from build123d import *

# Parameters (mm, degrees)
SKICA1_W                 = 150
SKICA1_H                 = 35
P_IDAT_VYSUNUT_M2_DEPTH  = 3
SKICA2_W                 = 6.5
SKICA2_H                 = 11.5
SKICA2_W_2               = 5
SKICA2_H_2               = 10
P_IDAT_VYSUNUT_M3_DEPTH  = 2
SKICA4_W                 = 20
SKICA4_H                 = 5
ODEBRAT_VYSUNUT_M1_DEPTH = 2
SKICA5_W                 = 150
SKICA5_H                 = 5.2
ODEBRAT_VYSUNUT_M3_DEPTH = 1
SKICA7_R                 = 2
ODEBRAT_VYSUNUT_M4_DEPTH = 5
SKICA8_W                 = 8
SKICA8_H                 = 6
P_IDAT_VYSUNUT_M4_DEPTH  = 30
ZAOBLIT1_R               = 1
SKICA9_W                 = 134
SKICA9_H                 = 1
P_IDAT_VYSUNUT_M5_DEPTH  = 4
ZAOBLIT2_R               = 1


with BuildPart() as part:
    # Skica1 → Přidat vysunutím2 (new body)
    with BuildSketch(Plane.XY):
        Rectangle(SKICA1_W, SKICA1_H)
    extrude(amount=P_IDAT_VYSUNUT_M2_DEPTH)

    # Skica2 → Přidat vysunutím3 (add)
    with BuildSketch(Plane.XY.offset(3)):
        with Locations((-22.5, 0)):
            Rectangle(SKICA2_W, SKICA2_H)
        with Locations((-22.5, 0)):
            Rectangle(SKICA2_W_2, SKICA2_H_2, mode=Mode.SUBTRACT)
        with Locations((12.5, 0)):
            Rectangle(SKICA2_W, SKICA2_H)
        with Locations((12.5, 0)):
            Rectangle(SKICA2_W_2, SKICA2_H_2, mode=Mode.SUBTRACT)
    extrude(amount=P_IDAT_VYSUNUT_M3_DEPTH)

    # Skica4 → Odebrat vysunutím1 (cut)
    with BuildSketch(Plane.XY.offset(3)):
        with Locations((-5, 0)):
            Rectangle(SKICA4_W, SKICA4_H)
    extrude(amount=-ODEBRAT_VYSUNUT_M1_DEPTH, mode=Mode.SUBTRACT)

    # Skica5 → Odebrat vysunutím3 (cut)
    with BuildSketch(Plane(origin=(0, 0, 0), x_dir=(-1, 0, 0), z_dir=(0, 0, -1))):
        Rectangle(SKICA5_W, SKICA5_H)
    extrude(amount=-ODEBRAT_VYSUNUT_M3_DEPTH, mode=Mode.SUBTRACT)

    # Skica7 → Odebrat vysunutím4 (cut, through all)
    with BuildSketch(Plane(origin=(0, 0, 1), x_dir=(-1, 0, 0), z_dir=(0, 0, -1))):
        with Locations((-50, 0)):
            Circle(SKICA7_R)
        with Locations((50, 0)):
            Circle(SKICA7_R)
    extrude(amount=-ODEBRAT_VYSUNUT_M4_DEPTH, mode=Mode.SUBTRACT)

    # Skica8 → Přidat vysunutím4 (add)
    with BuildSketch(Plane.XY.offset(3)):
        with Locations((71, 14.5)):
            Rectangle(SKICA8_W, SKICA8_H)
        with Locations((71, -14.5)):
            Rectangle(SKICA8_W, SKICA8_H)
        with Locations((-71, -14.5)):
            Rectangle(SKICA8_W, SKICA8_H)
        with Locations((-71, 14.5)):
            Rectangle(SKICA8_W, SKICA8_H)
    extrude(amount=P_IDAT_VYSUNUT_M4_DEPTH)

    # Zaoblit1
    zaoblit1_edges = [part.edges().sort_by_distance(p)[0] for p in [
        (75, -17.5, 16.5),
        (75, 17.5, 16.5),
        (-75, 17.5, 16.5),
        (-75, -17.5, 16.5),
    ]]
    fillet(zaoblit1_edges, radius=ZAOBLIT1_R)

    # Skica9 → Přidat vysunutím5 (add)
    with BuildSketch(Plane.XY.offset(3)):
        with Locations((0, 17)):
            Rectangle(SKICA9_W, SKICA9_H)
        with Locations((0, -17)):
            Rectangle(SKICA9_W, SKICA9_H)
    extrude(amount=P_IDAT_VYSUNUT_M5_DEPTH)

    # Zaoblit2
    zaoblit2_edges = [part.edges().sort_by_distance(p)[0] for p in [
        (67, 17, 7),
        (-67, 17, 7),
        (-67, -17, 7),
        (67, -17, 7),
    ]]
    fillet(zaoblit2_edges, radius=ZAOBLIT2_R)


solid = part.part
Input: part model. Units: mm. Frame: model coordinates. A direction names the side the tool comes from. Give positions to 0.01 mm unless a question says otherwise; leave off trailing zeros. Write each loop counter-clockwise with the first axis right and the second up, starting at its lowest first coordinate (ties: lowest second). Pieces come first, ordered by that corner, then holes. Notation, with made-up numbers: M -36,87 L 0,87 A17 ccw 0,99 Z; hole C -33,40.5 d1. An arc over 180 degrees is marked long. Write item = value, one per line. Start each with the question number.
1) Material intervals for line 1 along Y through (x, z) = (-50, 1.6); line 2 along X through (y, z) = (-15, 13); line 3 along Z through (x, y) = (-36.5, -16), sorted ascending. Write a range as [from, to].
2) Cut plane C-C on y = 0. Count the separate pieces of the cut face and the enclosed holes in it, then the cut area to 3 significant figures.
3) Draft query along X for faces 4 (the flat face through (67, -15, 18)), 5 (the flat face through (-71, 11.5, 18)), 6 (the cylindrical face through (52, 0, 2)). Return one class per face: +X half, -X half, draft (parallel to the pull), parting line (faces both ways), or undercut.
4) Cut plane A-A on z = 16. Return the cut outline in (x, y), then the cut area to 3 significant figures.
5) First-contact query: pin 1 Ø1 at (y, z) = (1, 4) entering from -X; pin 2 Ø10 at (x, y) = (34, 10) entering from +Z; pin 3 Ø10 at (y, z) = (-9.5, 26) entering from -X; pin 4 Ø5.5 at (x, y) = (12, 0.5) entering from +Z. Flat tips, straight axial feed; report the tip coordinate or a pass-through.
6) Cut plane B-B on x = 50. Return the cut outline in (y, z).
7) Reachability of faces 1 (the flat face through (71, -14, 33)), 2 (the flat face through (-1, 16.5, 5)), 3 (the flat face through (-25.4, 0.1, 5)) from +Z, -Z, +X, -X, +Y, -Y: full face, straight path, thin tool, end or side. Return the list, or none.
Solved:
q1.line_1 = [-17.5, -2], [2, 17.5]
q1.line_2 = [-75, -67], [67, 75]
q1.line_3 = [0, 3]
q2.separate_pieces = 4
q2.enclosed_holes = 0
q2.area = 250 mm2
q3.face_4 = undercut
q3.face_5 = draft
q3.face_6 = undercut
q4.outline = M -75,-16.5 A1 ccw -74,-17.5 L -67,-17.5 L -67,-11.5 L -75,-11.5 Z; M -75,11.5 L -67,11.5 L -67,17.5 L -74,17.5 A1 ccw -75,16.5 Z; M 67,-17.5 L 74,-17.5 A1 ccw 75,-16.5 L 75,-11.5 L 67,-11.5 Z; M 67,11.5 L 75,11.5 L 75,16.5 A1 ccw 74,17.5 L 67,17.5 Z
q4.area = 191 mm2
q5.pin_1 = -25.75
q5.pin_2 = 3
q5.pin_3 = -75
q5.pin_4 = 5
q6.outline = M -17.5,0 L -2.6,0 L -2.6,1 L -2,1 L -2,3 L -16.5,3 L -16.5,7 L -17.5,7 Z; M 2,1 L 2.6,1 L 2.6,0 L 17.5,0 L 17.5,7 L 16.5,7 L 16.5,3 L 2,3 Z
q7.face_1 = +Z, +X, -X, +Y, -Y
q7.face_2 = +Z
q7.face_3 = +Z, +X, -X
